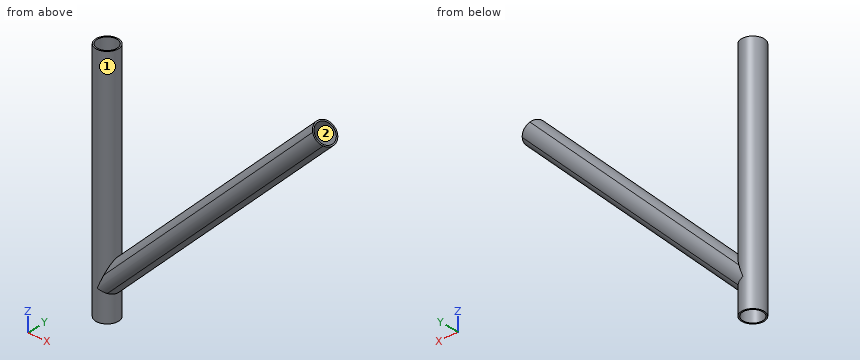
```python
from build123d import *

# Parameters (mm, degrees)
SKETCH1_R             = 9.525
SKETCH1_R_2           = 8.382
BOSS_EXTRUDE2_DEPTH   = 203.2
SWEEP_THIN1_START     = 17.960512242
SWEEP_THIN1_OUTLINE_R = 8.382
SWEEP_THIN1_DEPTH     = 261.968195874


# Read off the part's stored shape, not the designer's step: Sweep-Thin1
with BuildPart() as part:
    # Sketch1 → Boss-Extrude2 (new body)
    with BuildSketch(Plane.XY):
        with Locations(Location((0, 0, 0), (0, 0, 180))):
            Circle(SKETCH1_R)
        with Locations(Location((0, 0, 0), (0, 0, 180))):
            Circle(SKETCH1_R_2, mode=Mode.SUBTRACT)
    extrude(amount=BOSS_EXTRUDE2_DEPTH)

    # Sweep-Thin1 outline → Sweep-Thin1 (add)
    with BuildSketch(Plane(origin=(0, 0, 0), x_dir=(0.7071067811865474, 0, -0.7071067811865477), z_dir=(0.7071067811865476, 0, 0.7071067811865476)).offset(SWEEP_THIN1_START)):
        with BuildLine():
            ThreePointArc((-22.484132156, 8.382272238), (-27.48551224, 0.000176979), (-22.484443646, -8.382104131))
            ThreePointArc((-22.484443646, -8.382104131), (-16.812644927, -9.455581718), (-11.562434249, -7.056218747))
            ThreePointArc((-11.562434249, -7.056218747), (-8.435512242, 0), (-11.562434249, 7.056218747))
            ThreePointArc((-11.562434249, 7.056218747), (-16.812469239, 9.455560389), (-22.484132156, 8.382272238))
        make_face()
        with Locations((-17.960512242, 0)):
            Circle(SWEEP_THIN1_OUTLINE_R, mode=Mode.SUBTRACT)
    extrude(amount=SWEEP_THIN1_DEPTH)


solid = part.part
```
Design review of the part built by this model. Coordinates are the model's own, in mm. Face numbers are marked on the shaded views. Coordinates: 2 decimals unless noted, no trailing zeros. Loops run counter-clockwise (first coordinate to the right, second up) from the corner with the lowest first, then second, coordinate; pieces in that order, holes last. Notation, with made-up numbers: M 38,84.25 L 90,84.25 A20 cw 90,115.25 Z; hole C 47,77 d5. An arc over 180 degrees is marked long. One line per question, with ' | ' between items.
(1) For pin 1 Ø1.5 at (y, z) = (5.5, 156.5) entering from +X; pin 2 Ø5.5 at (x, y) = (-2.5, 1.5) entering from +Z; pin 3 Ø3 at (x, y) = (27.5, 4) entering from -Z, all flat-tipped, find the tip position at first contact; note any pin that passes through.
Filled in:
pin 1: stops at x = 143.12 | pin 2: stops at z = 39 | pin 3: stops at z = 38.94
(2) We need section B-B (z = 112). Count the separate pieces of the cut face and the enclosed holes in it, and give its area (3 significant figures).
Filled in:
separate pieces: 2 | enclosed holes: 2 | area: 155 mm^2
(3) We need section A-A (y = 0). Give the boundary of the cut face in (x, z) (3 decimals).
Filled in:
outline: M -9.525,0 L -8.382,0 L -8.382,203.2 L -9.525,203.2 Z; M -6.735,32.135 L -5.927,31.327 L 8.382,45.636 L 8.382,21.928 L 5.927,19.473 L 6.735,18.665 L 8.382,20.312 L 8.382,0 L 9.525,0 L 9.525,21.455 L 191.975,203.904 L 191.166,204.713 L 9.525,23.071 L 9.525,46.779 L 179.313,216.566 L 178.504,217.375 L 9.525,48.395 L 9.525,203.2 L 8.382,203.2 L 8.382,47.252 Z
(4) Draft analysis for pull direction X (two halves, no side actions). For the marked faces 1 and 2, state which applies: released by +X, released by -X, zero draft, split by the parting line, or undercut.
Filled in:
face 1: undercut | face 2: undercut
(5) Wall thickness on probe 1 along Y at (x, z) = (0, 73.5) (3 decimals); probe 2 along X at (y, z) = (1.5, 202); probe 3 along X at (y, z) = (0.25, 73): over which ranges is each line inside the solid? List them lowest first.
Filled in:
probe 1: y = -9.525 to -8.382, 8.382 to 9.525 | probe 2: x = -9.41 to -8.25, 8.25 to 9.41, 163.3 to 164.94, 188.26 to 189.9 | probe 3: x = -9.52 to -8.38, 8.38 to 9.52, 34.13 to 35.75, 59.45 to 61.07
